```python
from build123d import *

# Parameters (mm, degrees)
SKETCH1_W         = 1.651
SKETCH1_H         = 111.125
CHAMFER1_SIZE     = 1.27
SKETCH3_R         = 1.27
VENTHOLES_DEPTH   = 91.315461444
CIRPATTERN1_COUNT = 2
CIRPATTERN1_ANGLE = 90


with BuildPart() as part:
    # Sketch1 → Revolve1 (revolve)
    with BuildSketch(Plane(origin=(0, 0, 0), x_dir=(1, 0, 0), z_dir=(0, 1, 0))):
        with Locations((36.0045, 18.220863815)):
            Rectangle(SKETCH1_W, SKETCH1_H)
    revolve(axis=Axis((0, 0, 37.341636185), (0, 0, -1)))

    # Chamfer1
    chamfer1_edges = [part.edges().sort_by_distance(p)[0] for p in [
        (-35.179, 0, 37.341636185),
        (-35.179, 0, -73.783363815),
    ]]
    chamfer(chamfer1_edges, length=CHAMFER1_SIZE)

    # Sketch3 → ventholes (cut, symmetric)
    with BuildSketch(Plane(origin=(0, 0, 0), x_dir=(1, 0, 0), z_dir=(0, 1, 0))):
        with Locations(Location((0, 18.220863815, 0), (0, 0, 270))):
            Circle(SKETCH3_R)
    ventholes = extrude(amount=VENTHOLES_DEPTH, both=True, mode=Mode.SUBTRACT)

    # CirPattern1: ventholes ×2 about axis
    cirpattern1_axis = Axis((0, 0, 37.341636185), (0, 0, 1))
    for i in range(1, CIRPATTERN1_COUNT):
        add(ventholes.rotate(cirpattern1_axis, i * CIRPATTERN1_ANGLE / (CIRPATTERN1_COUNT - 1)), mode=Mode.SUBTRACT)


solid = part.part
```
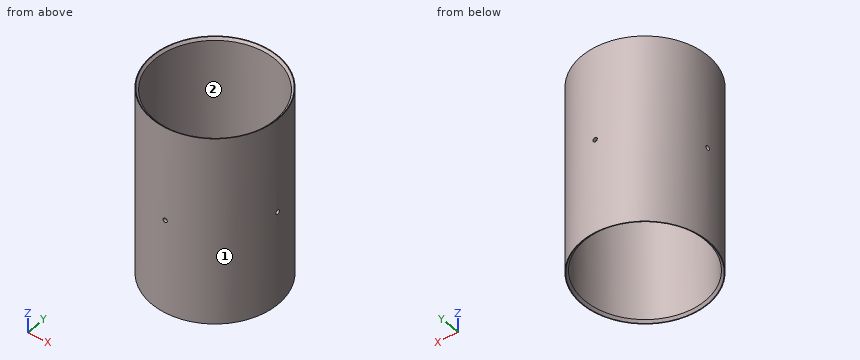
Part model, mm, in its own coordinate system. Face numbers are marked on the shaded views. Round coordinates to 2 decimals unless told otherwise and drop trailing zeros. Write each loop counter-clockwise with the first axis right and the second up, starting at its lowest first coordinate (ties: lowest second). Pieces come first, ordered by that corner, then holes.
Item 1: Two-plate mould, pull along X, no slides. Class the marked faces 1 and 2: +X half, -X half, draft (parallel to the pull), parting line (faces both ways), or undercut.
Results:
face 1: parting line
face 2: undercut
Item 2: Drop flat-ended pins along their axis: pin 1 Ø4 at (y, z) = (25, -34) entering from +X; pin 2 Ø10 at (x, z) = (26, -55) entering from +Y; pin 3 Ø6 at (x, z) = (4, 19.5) entering from +Y. Give the stop position or say it passes through.
Results:
pin 1: stops at x = 28.77
pin 2: stops at y = 30.26
pin 3: stops at y = 36.82
Item 3: Cut at C-C, the plane z = -25. Give the cut face in (x, y).
Results:
outline: circle Ø73.66 at (0, 0); hole circle Ø70.36 at (0, 0)
Item 4: Probe L1, parallel to X at y = 0, z = -1; L2, parallel to Y at x = 25, z = -40. List the from-to ranges inside material, lowest first.
Results:
L1: x = -36.83 to -35.18, 35.18 to 36.83
L2: y = -27.05 to -24.75, 24.75 to 27.05
Item 5: Cut at A-A, the plane y = 0. Give the cut face in (x, z).
Results:
outline: (-36.83, -73.78) - (-36.45, -73.78) - (-35.18, -72.51) - (-35.18, -19.49) - (-36.83, -19.49) - close; (-36.83, -16.95) - (-35.18, -16.95) - (-35.18, 36.07) - (-36.45, 37.34) - (-36.83, 37.34) - close; (35.18, -72.51) - (36.45, -73.78) - (36.83, -73.78) - (36.83, -19.49) - (35.18, -19.49) - close; (35.18, -16.95) - (36.83, -16.95) - (36.83, 37.34) - (36.45, 37.34) - (35.18, 36.07) - close
